Part model, mm, in its own coordinate system. Face numbers are marked on the shaded views. Coordinates: 2 decimals unless noted, no trailing zeros. Write each loop counter-clockwise with the first axis right and the second up, starting at its lowest first coordinate (ties: lowest second). Pieces come first, ordered by that corner, then holes. Notation, with made-up numbers: (23.5, 70) -> (54.5, 70) arc R15 cw to (54.5, 84) -> close; hole circle Ø4 at (89, 1). An arc over 180 degrees is marked (long way). Write item = value, one per line. Start each with the question number.
Q1. Band-saw the part on C-C, the plane z = 7.75. List the corners of the cut face in (x, y), plus the area to 3 significant figures.
Q2. Pin check, flat tips, straight feed: P1, Ø10, axis at x = 1.5, y = -13, coming from the -Z side; P2, Ø1, axis at y = 1, z = 9, coming from the -X side; P3, Ø4, axis at x = -17.5, z = 9.5, coming from the +Y side; P4, Ø3, axis at x = -8, z = 2.5, coming from the -Y side. Stop position of each tip, or through.
Q3. Band-saw the part on A-A, the plane y = 0. List the corners of the cut face in (x, z), plus the area to 3 significant figures.
Q4. Probe line 1 (Y direction, x = 0, z = 10.25); line 2 (Y direction, x = 0, z = 0.95); line 3 (X direction, y = -0.5, z = 11.25). List the from-to ranges inside material, lowest first.
Q5. Pull direction Y, two halves, no side cores. Call the marked faces 1, 2, 3 and 4: released by +Y, released by -Y, zero draft, split by the parting line, or undercut.
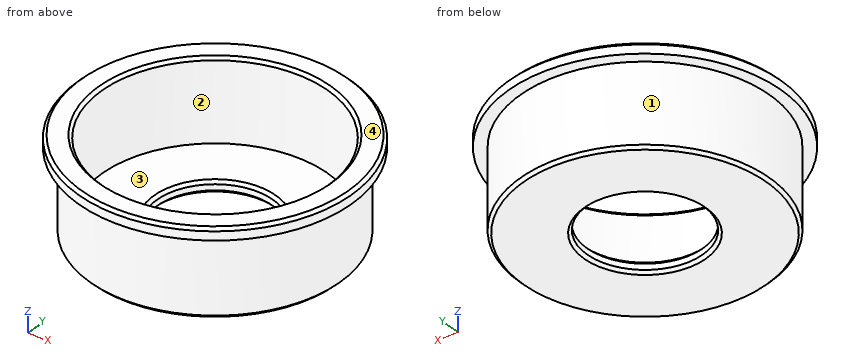
from build123d import *

# Parameters (mm, degrees)
F0_R     = 21.5
F0_R_2   = 10
F1_DEPTH = 2
F2_R     = 21.5
F2_R_2   = 19.5
F3_DEPTH = 12
F4_R     = 23.5
F4_R_2   = 21.5
F4_R_3   = 19.5
F5_DEPTH = 2
F6_SIZE  = 0.5
F7_SIZE  = 0.5
F8_SIZE  = 0.5


with BuildPart() as f1:
    # F0 (on Top) → F1 (new body)
    with BuildSketch(Plane.XY):
        Circle(F0_R)
        Circle(F0_R_2, mode=Mode.SUBTRACT)
    extrude(amount=F1_DEPTH)

    # F2 (on face) → F3 (join)
    with BuildSketch(Plane.XY.offset(2)):
        Circle(F2_R)
        Circle(F2_R_2, mode=Mode.SUBTRACT)
    extrude(amount=F3_DEPTH)

    # F4 (on face) → F5 (join)
    with BuildSketch(Plane.XY.offset(14)):
        Circle(F4_R)
        Circle(F4_R_2, mode=Mode.SUBTRACT)
        Circle(F4_R_2)
        Circle(F4_R_3, mode=Mode.SUBTRACT)
    extrude(amount=F5_DEPTH)

    # F6
    f6_edges = [f1.edges().sort_by_distance(p)[0] for p in [
        (-21.5, 0, 0),
    ]]
    chamfer(f6_edges, length=F6_SIZE)

    # F7
    f7_edges = [f1.edges().sort_by_distance(p)[0] for p in [
        (-10, 0, 2),
        (-10, 0, 0),
    ]]
    chamfer(f7_edges, length=F7_SIZE)

    # F8
    f8_edges = [f1.edges().sort_by_distance(p)[0] for p in [
        (-23.5, 0, 16),
        (-19.5, 0, 16),
    ]]
    chamfer(f8_edges, length=F8_SIZE)


solid = f1.part
Ans:
q1.outline = circle Ø43 at (0, 0); hole circle Ø39 at (0, 0)
q1.area = 258 mm2
q2.P1 = 0
q2.P2 = -21.49
q2.P3 = 14.9
q2.P4 = -20.49
q3.outline = (-23.5, 14) -> (-21.5, 14) -> (-21.5, 0.5) -> (-21, 0) -> (-10.5, 0) -> (-10, 0.5) -> (-10, 1.5) -> (-10.5, 2) -> (-19.5, 2) -> (-19.5, 15.5) -> (-20, 16) -> (-23, 16) -> (-23.5, 15.5) -> close; (10, 0.5) -> (10.5, 0) -> (21, 0) -> (21.5, 0.5) -> (21.5, 14) -> (23.5, 14) -> (23.5, 15.5) -> (23, 16) -> (20, 16) -> (19.5, 15.5) -> (19.5, 2) -> (10.5, 2) -> (10, 1.5) -> close
q3.area = 109 mm2
q4.line_1 = -21.5 to -19.5, 19.5 to 21.5
q4.line_2 = -21.5 to -10, 10 to 21.5
q4.line_3 = -21.49 to -19.49, 19.49 to 21.49
q5.face_1 = split by the parting line
q5.face_2 = undercut
q5.face_3 = undercut
q5.face_4 = zero draft
